The model under review builds one solid part; all positions refer to its coordinate system, in mm. A direction names the side the tool comes from. Give positions to 0.01 mm unless a question says otherwise; leave off trailing zeros. Loops run counter-clockwise (first coordinate to the right, second up) from the corner with the lowest first, then second, coordinate; pieces in that order, holes last. Notation, with made-up numbers: M 12,-19.75 L 67,-19.75 A13 cw 67,-11.75 Z; hole C -11.5,-10.75 d4. An arc over 180 degrees is marked long. One line per item, written item: value. Start each with the question number.
Q1. For pin 1 (1.1 mm diameter, centred on x = 29, y = 17, fed in from +Z); pin 2 (1 mm diameter, centred on x = 17.5, y = 11.5, fed in from -Z); pin 3 (4 mm diameter, centred on x = -6, y = 5.5, fed in from -Z); pin 4 (1.5 mm diameter, centred on x = 7.5, z = 19.5, fed in from -Y), all flat-tipped, find the tip position at first contact; note any pin that passes through.
Q2. We need section C-C on z = 21.5. Write out the cut boundary in (x, y), plus the area to 3 significant figures.
Q3. We need section B-B on x = 13. Write out the cut boundary in (y, z).
Q4. We need section A-A on z = 8. Write out the cut boundary in (x, y).
Q5. We need section D-D on y = 23. Write out the cut boundary in (x, z).
Q6. For faces 1 (the face through (30, 12, -29)), 2 (the face through (29.5, 10, -27)), 3 (the face through (29.5, 10, 0)), 4 (the face through (0, 4, -29)), 5 (the face through (-31.55, 6.08, -31.19)), list the 3-axis set-ups (+Z, -Z, +X, -X, +Y, -Y) from which the entire face can be reached by the end or side of a thin tool; tool diameter is ignored.
Q7. To check wall thickness, follow line 1 along X through (y, z) = (5.25, -19); line 2 along Z through (x, y) = (23.5, 2.5); line 3 along Z through (x, y) = (-5, 14.75). State the ranges of each line that lie inside material, in increasing order. Write a range as from..to.
Q8. Mouldability with a two-part tool opening along X and no side actions: class faces 6 (the face through (-29.5, 8, 0)), 7 (the face through (12.791, 12.002, 28.507)), 8 (the face through (-30, 12, -29)) as released by +X, released by -X, zero draft, split by the parting line, or undercut.
```python
from build123d import *

# Parameters (mm, degrees)
SKETCH1_W               = 59
SKETCH1_H               = 58
BOSS_EXTRUDE1_DEPTH     = 1
SKETCH2_W               = 59
SKETCH2_H               = 58
SKETCH2_W_2             = 57
SKETCH2_H_2             = 56
BOSS_EXTRUDE2_DEPTH     = 33
CUT_EXTRUDE1_DEPTH      = 1
CUT_EXTRUDE2_DEPTH      = 1
CUT_EXTRUDE3_DEPTH      = 1
SKETCH8_R               = 9.5
CUT_EXTRUDE4_DEPTH      = 1
SKETCH9_W               = 57
SKETCH9_H               = 26
CUT_EXTRUDE5_DEPTH      = 1
SKETCH11_W              = 3
SKETCH11_H              = 12
REVOLVE2_ANGLE          = 270
MIRROR2_COPY_1_SKETCH_W = 3
MIRROR2_COPY_1_SKETCH_H = 12
MIRROR2_COPY_1_ANGLE    = 270


with BuildPart() as part:
    # Sketch1 → Boss-Extrude1 (new body)
    with BuildSketch(Plane(origin=(0, 0, 0), x_dir=(1, 0, 0), z_dir=(0, 1, 0))):
        Rectangle(SKETCH1_W, SKETCH1_H)
    extrude(amount=BOSS_EXTRUDE1_DEPTH)

    # Sketch2 → Boss-Extrude2 (add)
    with BuildSketch(Plane(origin=(0, 1, 0), x_dir=(1, 0, 0), z_dir=(0, 1, 0))):
        Rectangle(SKETCH2_W, SKETCH2_H)
        Rectangle(SKETCH2_W_2, SKETCH2_H_2, mode=Mode.SUBTRACT)
    extrude(amount=BOSS_EXTRUDE2_DEPTH)

    # Sketch3 → Cut-Extrude1 (cut)
    with BuildSketch(Plane.ZY.offset(29.5)):
        Polygon((10.5, 8), (29, 8), (29, 34), (-29, 34), (-29, 8), (-10.5, 8), (-10.5, 20), (10.5, 20), align=None)
    extrude(amount=-CUT_EXTRUDE1_DEPTH, mode=Mode.SUBTRACT)

    # Sketch5 → Cut-Extrude2 (cut)
    with BuildSketch(Plane.XZ):
        Polygon((-21.5, 5.5), (-21.5, -5.5), (-5.5, -5.5), (-5.5, -15.5), (25.5, -15.5), (25.5, 15.5), (-5.5, 15.5), (-5.5, 5.5), align=None)
    extrude(amount=-CUT_EXTRUDE2_DEPTH, mode=Mode.SUBTRACT)

    # Sketch7 → Cut-Extrude3 (cut)
    with BuildSketch(Plane(origin=(29.5, 0, 0), x_dir=(0, 0, -1), z_dir=(1, 0, 0))):
        Polygon((29, 8), (10.5, 8), (10.5, 26), (-10.5, 26), (-10.5, 8), (-29, 8), (-29, 34), (29, 34), align=None)
    extrude(amount=-CUT_EXTRUDE3_DEPTH, mode=Mode.SUBTRACT)

    # Sketch8 → Cut-Extrude4 (cut)
    with BuildSketch(Plane.XY.offset(29)):
        with BuildLine():
            Line((22.5, 21.5), (28.5, 21.5))
            Line((28.5, 21.5), (28.5, 34))
            Line((28.5, 34), (-28.5, 34))
            Line((-28.5, 34), (-28.5, 21.5))
            Line((-28.5, 21.5), (-22.5, 21.5))
            ThreePointArc((-22.5, 21.5), (-13, 31), (-3.5, 21.5))
            Line((-3.5, 21.5), (3.5, 21.5))
            ThreePointArc((3.5, 21.5), (13, 31), (22.5, 21.5))
        make_face()
        with Locations((-13, 21.5)):
            Circle(SKETCH8_R)
        with Locations((13, 21.5)):
            Circle(SKETCH8_R)
    extrude(amount=-CUT_EXTRUDE4_DEPTH, mode=Mode.SUBTRACT)

    # Sketch9 → Cut-Extrude5 (cut)
    with BuildSketch(Plane(origin=(0, 0, -29), x_dir=(-1, 0, 0), z_dir=(0, 0, -1))):
        with Locations((0, 21)):
            Rectangle(SKETCH9_W, SKETCH9_H)
    extrude(amount=-CUT_EXTRUDE5_DEPTH, mode=Mode.SUBTRACT)

    # Sketch11 → Revolve2 (revolve)
    with BuildSketch(Plane.XY.offset(29)):
        with Locations((28, 6)):
            Rectangle(SKETCH11_W, SKETCH11_H)
    revolve2 = revolve(axis=Axis((29.5, 0, 29), (0, 1, 0)), revolution_arc=REVOLVE2_ANGLE)

    # Mirror1: Revolve2 across plane
    add(revolve2.mirror(Plane.XY))

    # Mirror2: Revolve2 across plane
    add(revolve2.mirror(Plane(origin=(0, 0, 0), x_dir=(0, 0, 1), z_dir=(1, 0, 0))))

    # Mirror2 copy 1 sketch → Mirror2 copy 1 (revolve)
    with BuildSketch(Plane(origin=(0, 0, -29), x_dir=(-1, 0, 0), z_dir=(0, 0, -1))):
        with Locations((28, 6)):
            Rectangle(MIRROR2_COPY_1_SKETCH_W, MIRROR2_COPY_1_SKETCH_H)
    revolve(axis=Axis((-29.5, 0, -29), (0, 1, 0)), revolution_arc=MIRROR2_COPY_1_ANGLE)


solid = part.part
```
Solved:
1. pin 1: z = 29
1. pin 2: z = 28
1. pin 3: z = -29
1. pin 4: y = 0
2. outline: M -29.5,0 L 29.5,0 L 29.5,8 L 28.5,8 L 28.5,1 L -28.5,1 L -28.5,8 L -29.5,8 Z
2. area: 73.0 mm2
3. outline: M 0,-29 L 8,-29 L 8,-28 L 1,-28 L 1,-15.5 L 0,-15.5 Z; M 0,15.5 L 1,15.5 L 1,28 L 12,28 L 12,29 L 0,29 Z
4. outline: M -29.5,0 L -5.5,0 L -5.5,1 L -28.5,1 L -28.5,20 L -29.5,20 Z; M 25.5,0 L 29.5,0 L 29.5,26 L 28.5,26 L 28.5,1 L 25.5,1 Z
5. outline: M 28.5,-10.5 L 29.5,-10.5 L 29.5,10.5 L 28.5,10.5 Z
6. face 1: -Z, +X, -X, +Y
6. face 2: +Y
6. face 3: +X, +Y, -Y
6. face 4: -Z, +Y, -Y
6. face 5: +Y, -Y
7. line 1: -29.5..-28.5, 28.5..29.5
7. line 2: -29..-28, 28..29
7. line 3: 28..29
8. face 6: released by -X
8. face 7: undercut
8. face 8: zero draft
